Solid Edge part; units mm, degrees
sketch "Sketch1" plane through (0, 0, 0) normal (0, 0, 1) x (1, 0, 0)
  circle A0 centre (0, 0) radius 1.5
extrude "Ajout_matière_1" add sketch "Sketch1" along normal mid plane 4.57
sketch "Sketch2" plane through (0, 0, 2.285) normal (0, 0, 1) x (1, 0, 0)
  circle A0 centre (0, 0) radius 1.75
extrude "Ajout_matière_2" add sketch "Sketch2" along normal blind 1.5
chamfer "Chanfrein_1" distance 1 angle 45 1 edges at (-1.75, 0, 3.785)
mirror "Mirror1" about plane through (0, 0, 0) normal (0, 0, 1) of "Ajout_matière_2"
chamfer "Chamfer1" distance 1 angle 45 1 edges at (-1.75, 0, -3.785)
sketch "Sketch3" plane through (0, 0, 0) normal (0, -1, 0) x (1, 0, 0)
  line L0 (-0.1251, 3.3533) -> (0.1251, 3.3533)
  line L1 (0.1251, 3.3533) -> (0.1251, 4.2167)
  line L2 (0.1251, 4.2167) -> (-0.1251, 4.2167)
  line L3 (-0.1251, 4.2167) -> (-0.1251, 3.3533)
extrude "Enlèvement_matière_1" cut sketch "Sketch3" along normal mid plane 157.2986
mirror "Mirror2" about plane through (0, 0, 0) normal (0, 0, 1) of "Enlèvement_matière_1"
properties material "Acrylique, haute performance"
Work out the finished part from the listing and answer in its coordinate system (mm). Give positions to 0.01 mm unless a question says otherwise; leave off trailing zeros. Loops run counter-clockwise (first coordinate to the right, second up) from the corner with the lowest first, then second, coordinate; pieces in that order, holes last. Notation, with made-up numbers: (57.5, 68) -> (96.5, 68) arc R17 cw to (96.5, 96) -> close; hole circle Ø11 at (31, 0). An arc over 180 degrees is marked (long way). Use CSV: the item, a comma, the result in double quotes.
1. Straight lines are drawn through the part: line 1 (Z direction, x = 0, y = 0.25); line 2 (X direction, y = 0.15, z = 3.5); line 3 (X direction, y = 0.05, z = -2). For each, find the intervals that lie inside material, in ascending order.
Found:
line 1,"-3.35 to 3.35"
line 2,"-1.02 to -0.13, 0.13 to 1.02"
line 3,"-1.5 to 1.5"
2. The part is cut by section C-C (z = 0.25). Write down the section's boundary in (x, y), then the cut area to 3 significant figures.
Found:
outline,"circle Ø3 at (0, 0)"
area,"7.07 mm^2"
3. The part is cut by section A-A (x = 0). Write down the section's boundary in (y, z) (3 decimals), then the cut area to 3 significant figures.
Found:
outline,"(-1.75, -2.785) -> (-1.182, -3.353) -> (1.182, -3.353) -> (1.75, -2.785) -> (1.75, -2.285) -> (1.5, -2.285) -> (1.5, 2.285) -> (1.75, 2.285) -> (1.75, 2.785) -> (1.182, 3.353) -> (-1.182, 3.353) -> (-1.75, 2.785) -> (-1.75, 2.285) -> (-1.5, 2.285) -> (-1.5, -2.285) -> (-1.75, -2.285) -> close"
area,"20.5 mm^2"
4. The mould has two halves that part along Z. Classify faces 1 (the cylindrical face through (-1.5, 0.07, 0.03)), 2 (the cylindrical face through (1.617, -0.67, -2.532)): +Z half, -Z half, draft (parallel to the pull), parting line (faces both ways), or undercut.
Found:
face 1,"undercut"
face 2,"draft"
5. The part is cut by section B-B (y = 0). Write down the section's boundary in (x, z) (3 decimals), then the cut area to 3 significant figures.
Found:
outline,"(-1.75, -2.785) -> (-0.75, -3.785) -> (-0.125, -3.785) -> (-0.125, -3.353) -> (0.125, -3.353) -> (0.125, -3.785) -> (0.75, -3.785) -> (1.75, -2.785) -> (1.75, -2.285) -> (1.5, -2.285) -> (1.5, 2.285) -> (1.75, 2.285) -> (1.75, 2.785) -> (0.75, 3.785) -> (0.125, 3.785) -> (0.125, 3.353) -> (-0.125, 3.353) -> (-0.125, 3.785) -> (-0.75, 3.785) -> (-1.75, 2.785) -> (-1.75, 2.285) -> (-1.5, 2.285) -> (-1.5, -2.285) -> (-1.75, -2.285) -> close"
area,"22.0 mm^2"
6. Flat-ended cylindrical pins translate along their axes: pin 1 Ø2 at (x, y) = (0, -0.5) entering from -Z (3 decimals); pin 2 Ø0.5 at (y, z) = (0, 3.5) entering from -X (3 decimals). Find the tip coordinate at first contact, or state that the pin passes through.
Found:
pin 1,"z = -3.785"
pin 2,"x = -1.285"
